```python
from build123d import *

# Parameters (mm, degrees)
SKETCH1_R      = 3.175
EXTRUDE1_DEPTH = 82.55
SKETCH2_W      = 38.1
SKETCH2_H      = 152.4
EXTRUDE2_DEPTH = 39.1


with BuildPart() as part:
    # Sketch1 → Extrude1 (new body, symmetric)
    with BuildSketch(Plane(origin=(0, 0, 0), x_dir=(1, 0, 0), z_dir=(0, 1, 0))):
        with BuildLine():
            Line((-19.05, -25.4), (19.05, -25.4))
            Line((19.05, -25.4), (19.05, 0))
            ThreePointArc((19.05, 0), (0, 19.05), (-19.05, 0))
            Line((-19.05, 0), (-19.05, -25.4))
        make_face()
        with Locations(Location((0, 0, 0), (0, 0, 270))):  # turned: the seam where the file's is
            Circle(SKETCH1_R, mode=Mode.SUBTRACT)
    extrude(amount=EXTRUDE1_DEPTH, both=True)

    # Sketch2 → Extrude2 (cut, through all)
    with BuildSketch(Plane(origin=(19.05, 0, 0), x_dir=(0, 0, -1), z_dir=(1, 0, 0))):
        Rectangle(SKETCH2_W, SKETCH2_H)
    extrude(amount=-EXTRUDE2_DEPTH, mode=Mode.SUBTRACT)


solid = part.part
```
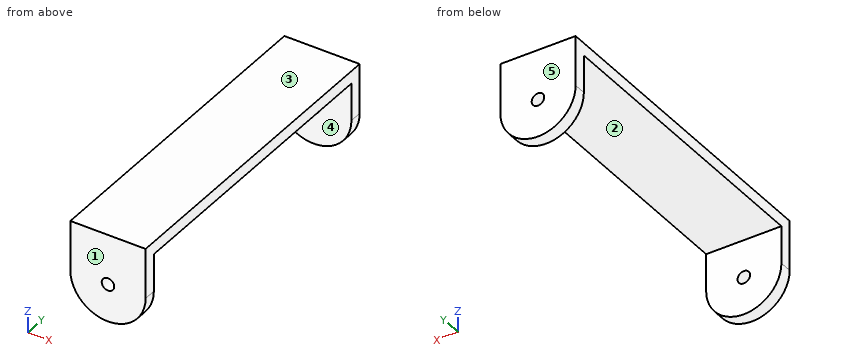
Can you work these out from the model? Positions are in its coordinate system, mm. Face numbers are marked on the shaded views. A direction names the side the tool comes from. Give positions to 0.01 mm unless a question says otherwise; leave off trailing zeros. Write each loop counter-clockwise with the first axis right and the second up, starting at its lowest first coordinate (ties: lowest second). Pieces come first, ordered by that corner, then holes. Notation, with made-up numbers: (67.5, -9) -> (98.5, -9) arc R17 cw to (98.5, 18) -> close; hole circle Ø7 at (85.25, 57.25). An arc over 180 degrees is marked (long way). Write item = value, one per line.
(1) For the marked faces 1 and 2, which set-ups out of +Z, -Z, +X, -X, +Y, -Y let a thin tool reach every point of the face, with its end or its side?
Worked out:
face_1 = +Z, -Z, +X, -X, -Y
face_2 = -Z, +X, -X
(2) I need wall thicknesses on probe 1 along Y at (x, z) = (-11, -0.5); probe 2 along Z at (x, y) = (0, 77) (3 decimals); probe 3 along Z at (x, y) = (17.5, 71). Which ranges of each line are inside material? Lowest first, please. Write a range as from..to.
Worked out:
probe_1 = -82.55..-76.2, 76.2..82.55
probe_2 = -19.05..-3.175, 3.175..25.4
probe_3 = 19.05..25.4
(3) Suppose I cut it at C-C on x = 13.5. Write out the boundary of the cut face in (y, z).
Worked out:
outline = (-82.55, -13.44) -> (-76.2, -13.44) -> (-76.2, 19.05) -> (76.2, 19.05) -> (76.2, -13.44) -> (82.55, -13.44) -> (82.55, 25.4) -> (-82.55, 25.4) -> close
(4) Suppose I cut it at B-B on x = 0. Write out the boundary of the cut face in (y, z) (3 decimals).
Worked out:
outline = (-82.55, -19.05) -> (-76.2, -19.05) -> (-76.2, -3.175) -> (-82.55, -3.175) -> close; (-82.55, 3.175) -> (-76.2, 3.175) -> (-76.2, 19.05) -> (76.2, 19.05) -> (76.2, 3.175) -> (82.55, 3.175) -> (82.55, 25.4) -> (-82.55, 25.4) -> close; (76.2, -19.05) -> (82.55, -19.05) -> (82.55, -3.175) -> (76.2, -3.175) -> close
(5) Suppose I cut it at D-D on y = 0. Write out the boundary of the cut face in (x, z), then the cut area to 3 significant figures.
Worked out:
outline = (-19.05, 19.05) -> (19.05, 19.05) -> (19.05, 25.4) -> (-19.05, 25.4) -> close
area = 242 mm^2
(6) Suppose I cut it at A-A on z = 7. Write out the boundary of the cut face in (x, y), then the cut area to 3 significant figures.
Worked out:
outline = (-19.05, -82.55) -> (19.05, -82.55) -> (19.05, -76.2) -> (-19.05, -76.2) -> close; (-19.05, 76.2) -> (19.05, 76.2) -> (19.05, 82.55) -> (-19.05, 82.55) -> close
area = 484 mm^2
(7) Thinking about a two-plate mould opening in Y: for the marked faces 3, 4 and 5, which applies, released by +Y, released by -Y, zero draft, split by the parting line, or undercut?
Worked out:
face_3 = zero draft
face_4 = undercut
face_5 = released by +Y
